Check sheet for the modelled part. Datum: model origin and axes. Units: mm. Round coordinates to 2 decimals unless told otherwise and drop trailing zeros. Order: outer loops, then holes, each group sorted by start corner. A loop starts at its lowest first (then second) coordinate and runs counter-clockwise, first axis right, second up.
Q1. Depth check by flat-ended pin: P1, Ø2.5, axis at y = 37.5, z = 2.5, coming from the -X side; P2, Ø2.5, axis at y = 56.5, z = 3.5, coming from the -X side; P3, Ø1.5, axis at x = 18, z = 2.5, coming from the -Y side. Enter the tip coordinate at first touch or a pass-through.
Q2. Mould release check, pull along X, two halves, no side actions. Record for faces 1 (the flat face through (35, 55, 2)), 2 (the flat face through (112.464, 60.381, 2.535)), 3 (the flat face through (72, 0, 2)): +X half, -X half, draft (parallel to the pull), parting line (faces both ways), or undercut.
Q3. Cross-section at B-B on x = 59.5. Record the cut outline in (y, z).
Q4. Scan lines: probe 1 along Y at (x, z) = (20, 3.55); probe 2 along X at (y, z) = (49.5, 4.1); probe 3 along Y at (x, z) = (13, 2.5). Record each from-to range of solid material in increasing order.
Q5. Cross-section at C-C on y = 34.5. Record the cut outline in (x, z), then the cut area to 3 significant figures.
Q6. Cross-section at A-A on x = 15. Record the cut outline in (y, z), then the cut area to 3 significant figures.
Q7. Cross-section at D-D on y = 105. Record the cut outline in (x, z).
from build123d import *

# Parameters (mm, degrees)
F1_DEPTH  = 5
F3_DEPTH  = 25
F5_DEPTH  = 5
F7_DEPTH  = 5
F9_DEPTH  = 5
F11_DEPTH = 5
F13_DEPTH = 5
F15_DEPTH = 5
F17_DEPTH = 5


with BuildPart() as f1:
    # F0 (on Top) → F1 (new body)
    with BuildSketch(Plane.XY):
        Polygon((120, 120), (0, 120), (0, 60), (35, 60), (35, 50), (25, 50), (25, 0), (120, 0), align=None)
    extrude(amount=F1_DEPTH)

    # F2 (on face) → F3 (cut)
    with BuildSketch(Plane.XY.offset(5)):
        Polygon((5, 115), (5, 65), (40, 65), (40, 45), (30, 45), (30, 5), (115, 5), (115, 115), align=None)
    extrude(amount=-F3_DEPTH, mode=Mode.SUBTRACT)

    # F4 (on face) → F5 (join)
    with BuildSketch(Plane.XY.offset(5)):
        Polygon((115, 8.5355339059), (8.5355339059, 115), (5, 115), (5, 111.4644660941), (111.4644660941, 5), (115, 5), align=None)
    extrude(amount=-F5_DEPTH)

    # F6 (on face) → F7 (join)
    with BuildSketch(Plane.XY.offset(5)):
        Polygon((70.3746479557, 53.1608859502), (115, 110.9113415369), (115, 115), (111.8405820967, 115), (66.8101764751, 56.7253574308), align=None)
        Polygon((67.2923876275, 49.1720784666), (70.3746479557, 53.1608859502), (66.8101764751, 56.7253574308), (63.7279161468, 52.7365499472), align=None)
        Polygon((33.1594179033, 5), (67.2923876275, 49.1720784666), (63.7279161468, 52.7365499472), (30, 9.0886584631), (30, 5), align=None)
    extrude(amount=-F7_DEPTH)

    # F8 (on face) → F9 (join)
    with BuildSketch(Plane.XY.offset(5)):
        Polygon((46.2973559623, 77.2381779437), (49.8618274429, 73.673706463), (81.7957815396, 115), (75.4769457331, 115), align=None)
        Polygon((43.215095634, 73.24937046), (46.7795671147, 69.6848989794), (49.8618274429, 73.673706463), (46.2973559623, 77.2381779437), align=None)
        Polygon((40, 65), (40, 60.9113415369), (46.7795671147, 69.6848989794), (43.215095634, 73.24937046), (36.8405820967, 65), align=None)
    extrude(amount=-F9_DEPTH)

    # F10 (on face) → F11 (join)
    with BuildSketch(Plane.XY.offset(5)):
        Polygon((25.9828204872, 97.5527134187), (29.5575639886, 93.9779699173), (45.1164897233, 115), (38.8959899157, 115), align=None)
        Polygon((22.9752933056, 93.4891727885), (26.550036807, 89.914429287), (29.5575639886, 93.9779699173), (25.9828204872, 97.5527134187), align=None)
        Polygon((5, 65), (8.1102499038, 65), (26.550036807, 89.914429287), (22.9752933056, 93.4891727885), (5, 69.2023317134), align=None)
    extrude(amount=-F11_DEPTH)

    # F12 (on face) → F13 (join)
    with BuildSketch(Plane.XY.offset(5)):
        Polygon((30, 45), (30, 41.4644660941), (44.1125315315, 27.3519345626), (47.1947918597, 31.3407420462), (33.5355339059, 45), align=None)
        Polygon((47.1947918597, 31.3407420462), (44.1125315315, 27.3519345626), (47.6770030121, 23.787463082), (50.7592633403, 27.7762705656), align=None)
        Polygon((50.7592633403, 27.7762705656), (47.6770030121, 23.787463082), (66.4644660941, 5), (73.5355339059, 5), align=None)
    extrude(amount=-F13_DEPTH)

    # F14 (on face) → F15 (join)
    with BuildSketch(Plane.XY.offset(5)):
        Polygon((52.1875575351, 115), (45.1164897233, 115), (62.2429008057, 97.8735889176), (65.325161134, 101.8623964012), align=None)
        Polygon((65.325161134, 101.8623964012), (62.2429008057, 97.8735889176), (65.8073722864, 94.3091174369), (68.8896326146, 98.2979249205), align=None)
        Polygon((68.8896326146, 98.2979249205), (65.8073722864, 94.3091174369), (82.7557213186, 77.3607684047), (85.8379816468, 81.3495758883), align=None)
        Polygon((89.4024531274, 77.7851044077), (86.3201927992, 73.7962969241), (115, 45.1164897233), (115, 52.1875575351), align=None)
        Polygon((85.8379816468, 81.3495758883), (82.7557213186, 77.3607684047), (86.3201927992, 73.7962969241), (89.4024531274, 77.7851044077), align=None)
    extrude(amount=-F15_DEPTH)

    # F16 (on face) → F17 (join)
    with BuildSketch(Plane.XY.offset(5)):
        Polygon((115, 71.8401578906), (106.4334818964, 60.7540756388), (109.997953377, 57.1896041582), (115, 63.6628409644), align=None)
        Polygon((106.4334818964, 60.7540756388), (103.3512215681, 56.7652681552), (106.9156930487, 53.2007966745), (109.997953377, 57.1896041582), align=None)
        Polygon((103.3512215681, 56.7652681552), (87.4056767246, 36.1298571813), (90.9701482053, 32.5653857007), (106.9156930487, 53.2007966745), align=None)
        Polygon((87.4056767246, 36.1298571813), (84.3234163964, 32.1410496977), (87.887887877, 28.576578217), (90.9701482053, 32.5653857007), align=None)
        Polygon((84.3234163964, 32.1410496977), (67.7902921093, 10.7452417967), (71.3547635899, 7.180770316), (87.887887877, 28.576578217), align=None)
    extrude(amount=-F17_DEPTH)


solid = f1.part
Results found:
1. P1: stops at x = 25
1. P2: stops at x = 35
1. P3: stops at y = 60
2. face 1: -X half
2. face 2: undercut
2. face 3: draft
3. outline: (0, 0) - (5, 0) - (5, 5) - (0, 5) - close; (11.96, 0) - (19.04, 0) - (19.04, 5) - (11.96, 5) - close; (39.09, 0) - (47.27, 0) - (47.27, 5) - (39.09, 5) - close; (56.96, 0) - (64.04, 0) - (64.04, 5) - (56.96, 5) - close; (86.15, 0) - (94.32, 0) - (94.32, 5) - (86.15, 5) - close; (100.62, 0) - (107.69, 0) - (107.69, 5) - (100.62, 5) - close; (115, 0) - (120, 0) - (120, 5) - (115, 5) - close
4. probe 1: y = 60 to 65, 81.06 to 89.47, 96.46 to 103.54, 115 to 120
4. probe 2: x = 25 to 40, 61.23 to 74.04, 97.74 to 104.06, 110.62 to 120
4. probe 3: y = 60 to 65, 71.61 to 80.01, 103.46 to 110.54, 115 to 120
5. outline: (25, 0) - (30, 0) - (30, 5) - (25, 5) - close; (36.96, 0) - (44.04, 0) - (44.04, 5) - (36.96, 5) - close; (49.64, 0) - (55.95, 0) - (55.95, 5) - (49.64, 5) - close; (81.96, 0) - (92.47, 0) - (92.47, 5) - (81.96, 5) - close; (115, 0) - (120, 0) - (120, 5) - (115, 5) - close
5. area: 169 mm2
6. outline: (60, 0) - (65, 0) - (65, 5) - (60, 5) - close; (74.31, 0) - (82.71, 0) - (82.71, 5) - (74.31, 5) - close; (101.46, 0) - (108.54, 0) - (108.54, 5) - (101.46, 5) - close; (115, 0) - (120, 0) - (120, 5) - (115, 5) - close
6. area: 127 mm2
7. outline: (0, 0) - (5, 0) - (5, 5) - (0, 5) - close; (11.46, 0) - (18.54, 0) - (18.54, 5) - (11.46, 5) - close; (31.49, 0) - (37.72, 0) - (37.72, 5) - (31.49, 5) - close; (55.12, 0) - (62.19, 0) - (62.19, 5) - (55.12, 5) - close; (67.75, 0) - (74.07, 0) - (74.07, 5) - (67.75, 5) - close; (104.11, 0) - (110.43, 0) - (110.43, 5) - (104.11, 5) - close; (115, 0) - (120, 0) - (120, 5) - (115, 5) - close
